Work out the finished part from the listing and answer in its coordinate system (mm). Face numbers are marked on the shaded views. A direction names the side the tool comes from. Coordinates: 2 decimals unless noted, no trailing zeros. Loops run counter-clockwise (first coordinate to the right, second up) from the corner with the lowest first, then second, coordinate; pieces in that order, holes last. Notation, with made-up numbers: (60, 53.5) -> (118, 53.5) arc R30 cw to (118, 90.5) -> close; hole circle Ø9 at (-19.75, 32.25). An arc over 180 degrees is marked (long way). Answer as CSV lines item,"result".
```python
from build123d import *

# Parameters (mm, degrees)
SKETCH2_R           = 24
SKETCH2_R_2         = 21
BOSS_EXTRUDE1_DEPTH = 50
CUT_EXTRUDE1_DEPTH  = 57


with BuildPart() as part:
    # Sketch2 → Boss-Extrude1 (new body, symmetric)
    with BuildSketch(Plane.XY):
        with BuildLine():
            Line((29.933259094, 20), (370.066740906, 20))
            ThreePointArc((370.066740906, 20), (436, 0), (370.066740906, -20))
            Line((370.066740906, -20), (29.933259094, -20))
            ThreePointArc((29.933259094, -20), (-36, 0), (29.933259094, 20))
        make_face()
        Circle(SKETCH2_R, mode=Mode.SUBTRACT)
        with Locations((400, 0)):
            Circle(SKETCH2_R_2, mode=Mode.SUBTRACT)
    extrude(amount=BOSS_EXTRUDE1_DEPTH, both=True)

    # Sketch3 → Cut-Extrude1 (cut, through all)
    with BuildSketch(Plane(origin=(0, 20, 0), x_dir=(1, 0, 0), z_dir=(0, 1, 0))):
        with BuildLine():
            Line((95, 25), (285, 25))
            ThreePointArc((285, 25), (295.606601718, 20.606601718), (300, 10))
            Line((300, 10), (300, -10))
            ThreePointArc((300, -10), (295.606601718, -20.606601718), (285, -25))
            Line((285, -25), (95, -25))
            ThreePointArc((95, -25), (84.393398282, -20.606601718), (80, -10))
            Line((80, -10), (80, 10))
            ThreePointArc((80, 10), (84.393398282, 20.606601718), (95, 25))
        make_face()
    extrude(amount=-CUT_EXTRUDE1_DEPTH, mode=Mode.SUBTRACT)


solid = part.part
```
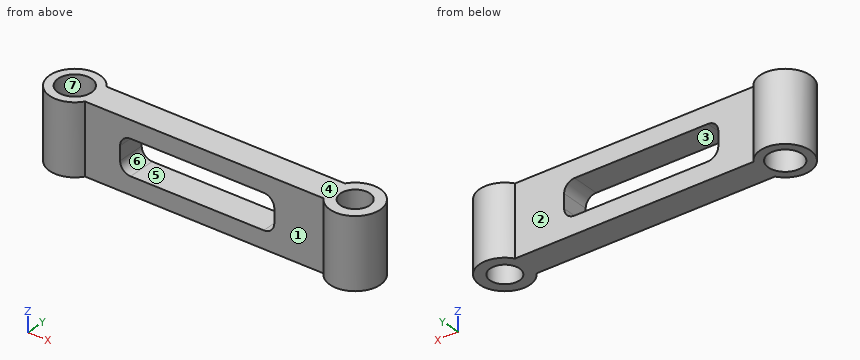
(1) A cutting plane is placed at C-C, the plane y = 8. Write down the section's boundary in (x, z).
Computed values:
outline,"(-35.1, -50) -> (-22.63, -50) -> (-22.63, 50) -> (-35.1, 50) -> close; (22.63, -50) -> (380.58, -50) -> (380.58, 50) -> (22.63, 50) -> close; (419.42, -50) -> (435.1, -50) -> (435.1, 50) -> (419.42, 50) -> close; hole (80, -10) arc R15 ccw to (95, -25) -> (285, -25) arc R15 ccw to (300, -10) -> (300, 10) arc R15 ccw to (285, 25) -> (95, 25) arc R15 ccw to (80, 10) -> close"
(2) Consider line 1 along Y through (x, z) = (0, 0); line 2 along Y through (x, z) = (400, 3); line 3 along Z through (x, y) = (194.5, -2.5). Determine where each line is inside the solid, lowest interval first.
Computed values:
line 1,"-36 to -24, 24 to 36"
line 2,"-36 to -21, 21 to 36"
line 3,"-50 to -25, 25 to 50"
(3) For a pull along Z with two mould halves and no side action, classify the marked faces 4, 5, 6 and 7 as pulls with the +Z half, pulls with the -Z half, needs draft (parallel to the pull), parting line crosses it, or undercut.
Computed values:
face 4,"pulls with the +Z half"
face 5,"undercut"
face 6,"undercut"
face 7,"needs draft"
(4) Which of the six approach directions +Z, -Z, +X, -X, +Y, -Y give full straight-line access (tool end or side, diameter ignored) to the marked faces 1, 2 and 3?
Computed values:
face 1,"+Z, -Z, -Y"
face 2,"+Z, -Z, +Y"
face 3,"+Y, -Y"
(5) Flat-ended cylindrical pins translate along their axes: pin 1 Ø5 at (y, z) = (3, 2.5) entering from -X; pin 2 Ø4 at (x, z) = (21, 34.5) entering from -Y; pin 3 Ø6 at (y, z) = (23.5, -10) entering from +X. Find the tip coordinate at first contact, or state that the pin passes through.
Computed values:
pin 1,"x = -36"
pin 2,"y = -30.58"
pin 3,"x = 429.59"
(6) A cutting plane is placed at B-B, the plane x = 400. Write down the section's boundary in (y, z).
Computed values:
outline,"(-36, -50) -> (-21, -50) -> (-21, 50) -> (-36, 50) -> close; (21, -50) -> (36, -50) -> (36, 50) -> (21, 50) -> close"
(7) A cutting plane is placed at A-A, the plane z = 2.5. Write down the section's boundary in (x, y), and give its area (3 significant figures).
Computed values:
outline,"(29.93, -20) -> (80, -20) -> (80, 20) -> (29.93, 20) arc R36 ccw (long way) to start; (300, -20) -> (370.07, -20) arc R36 ccw (long way) to (370.07, 20) -> (300, 20) -> close; hole circle Ø48 at (0, 0); hole circle Ø42 at (400, 0)"
area,"9,420 mm2"
(8) A cutting plane is placed at D-D, the plane x = 0. Write down the section's boundary in (y, z).
Computed values:
outline,"(-36, -50) -> (-24, -50) -> (-24, 50) -> (-36, 50) -> close; (24, -50) -> (36, -50) -> (36, 50) -> (24, 50) -> close"
